from build123d import *

# Parameters (mm, degrees)
ESBO_O1_W                  = 90
ESBO_O1_H                  = 90
ESBO_O1_W_2                = 84
ESBO_O1_H_2                = 84
EXTRUS_O_FINA2_DEPTH       = 45
CORTE_EXTRUS_O1_DEPTH      = 78.942286341
CORTE_EXTRUS_O1_DEPTH_BACK = 78.942286341
ESBO_O5_W                  = 3
ESBO_O5_H                  = 84
ESBO_O7_R                  = 45
ESBO_O7_R_2                = 42
EXTRUS_O_FINA4_DEPTH       = 45
CORTE_EXTRUS_O2_DEPTH      = 111.227038425
CORTE_EXTRUS_O2_DEPTH_BACK = 111.227038425
ESBO_O9_W                  = 3
ESBO_O9_H                  = 45
RESSALTO_EXTRUS_O1_DEPTH   = 45
ESBO_O10_W                 = 3
ESBO_O10_H                 = 90
RESSALTO_EXTRUS_O2_DEPTH   = 45
ESBO_O11_W                 = 3
ESBO_O11_H                 = 90
RESSALTO_EXTRUS_O3_DEPTH   = 45
CORTE_EXTRUS_O4_DEPTH      = 78.942286341
CORTE_EXTRUS_O4_DEPTH_BACK = 78.942286341
CORTE_EXTRUS_O5_DEPTH      = 78.942286341
CORTE_EXTRUS_O5_DEPTH_BACK = 78.942286341
ESBO_O14_R                 = 42
CORTE_EXTRUS_O6_DEPTH      = 78.942286341
CORTE_EXTRUS_O6_DEPTH_BACK = 78.942286341
ESBO_O16_W                 = 84
ESBO_O16_H                 = 42
CORTE_EXTRUS_O8_DEPTH      = 78.942286341


with BuildPart() as part:
    # Esboço1 → Extrusão-Fina2 (new, symmetric)
    with BuildSketch(Plane(origin=(0, 0, 0), x_dir=(0, 0, -1), z_dir=(1, 0, 0))):
        Rectangle(ESBO_O1_W, ESBO_O1_H)
        Rectangle(ESBO_O1_W_2, ESBO_O1_H_2, mode=Mode.SUBTRACT)
    extrude(amount=EXTRUS_O_FINA2_DEPTH, both=True)

    # Esboço5 → Corte-extrusão1 (cut, two sides: drawn at the far end of the back side and taken through both)
    with BuildSketch(Plane(origin=(0, 0, 0), x_dir=(0, 0, -1), z_dir=(1, 0, 0)).offset(-CORTE_EXTRUS_O1_DEPTH_BACK)):
        with Locations((-43.5, 0)):
            Rectangle(ESBO_O5_W, ESBO_O5_H)
    extrude(amount=CORTE_EXTRUS_O1_DEPTH + CORTE_EXTRUS_O1_DEPTH_BACK, mode=Mode.SUBTRACT)

    # Esboço7 → Extrusão-Fina4 (add, symmetric)
    with BuildSketch(Plane(origin=(0, 0, 0), x_dir=(0, 0, -1), z_dir=(1, 0, 0))):
        with Locations((-45, 0)):
            Circle(ESBO_O7_R)
        with Locations((-45, 0)):
            Circle(ESBO_O7_R_2, mode=Mode.SUBTRACT)
    extrude(amount=EXTRUS_O_FINA4_DEPTH, both=True)

    # Esboço8 → Corte-extrusão2 (cut, two sides: drawn at the far end of the back side and taken through both)
    with BuildSketch(Plane(origin=(0, 0, 0), x_dir=(0, 0, -1), z_dir=(1, 0, 0)).offset(-CORTE_EXTRUS_O2_DEPTH_BACK)):
        Polygon((-45, -45), (-29.921616549, -39.200030007), (-3, 0), (-3, 45), (-95.371690307, 45), (-95.371690307, -45), align=None)
    extrude(amount=CORTE_EXTRUS_O2_DEPTH + CORTE_EXTRUS_O2_DEPTH_BACK, mode=Mode.SUBTRACT)

    # Esboço9 → Ressalto-extrusão1 (add, symmetric)
    with BuildSketch(Plane(origin=(0, 0, 0), x_dir=(0, 0, -1), z_dir=(1, 0, 0))):
        with Locations((-1.5, 22.5)):
            Rectangle(ESBO_O9_W, ESBO_O9_H)
    extrude(amount=RESSALTO_EXTRUS_O1_DEPTH, both=True)

    # Esboço10 → Ressalto-extrusão2 (add, symmetric)
    with BuildSketch(Plane(origin=(0, 0, 0), x_dir=(1, 0, 0), z_dir=(0, 1, 0))):
        with Locations((-43.5, 0)):
            Rectangle(ESBO_O10_W, ESBO_O10_H)
    extrude(amount=RESSALTO_EXTRUS_O2_DEPTH, both=True)

    # Esboço11 → Ressalto-extrusão3 (add, symmetric)
    with BuildSketch(Plane(origin=(0, 0, 0), x_dir=(1, 0, 0), z_dir=(0, 1, 0))):
        with Locations((43.5, 0)):
            Rectangle(ESBO_O11_W, ESBO_O11_H)
    extrude(amount=RESSALTO_EXTRUS_O3_DEPTH, both=True)

    # Esboço13 → Corte-extrusão4 (cut, two sides: drawn at the far end of the back side and taken through both)
    with BuildSketch(Plane(origin=(0, 0, 0), x_dir=(0, 0, -1), z_dir=(1, 0, 0)).offset(-CORTE_EXTRUS_O4_DEPTH_BACK)):
        Polygon((-3, 0), (-3, 45), (-45, 45), (-45, -45), align=None)
    extrude(amount=CORTE_EXTRUS_O4_DEPTH + CORTE_EXTRUS_O4_DEPTH_BACK, mode=Mode.SUBTRACT)

    # Esboço14 → Corte-extrusão5 (cut, two sides: drawn at the far end of the back side and taken through both)
    with BuildSketch(Plane(origin=(0, 0, 0), x_dir=(0, 0, -1), z_dir=(1, 0, 0)).offset(-CORTE_EXTRUS_O5_DEPTH_BACK)):
        with Locations((-45, 0)):
            Circle(ESBO_O14_R)
    extrude(amount=CORTE_EXTRUS_O5_DEPTH + CORTE_EXTRUS_O5_DEPTH_BACK, mode=Mode.SUBTRACT)

    # Esboço15 → Corte-extrusão6 (cut, two sides: drawn at the far end of the back side and taken through both)
    with BuildSketch(Plane(origin=(0, 0, 0), x_dir=(0, 0, -1), z_dir=(1, 0, 0)).offset(-CORTE_EXTRUS_O6_DEPTH_BACK)):
        Polygon((-45, -45), (-29.921616549, -39.200030007), (-45.529383671, 1.376024306), align=None)
    extrude(amount=CORTE_EXTRUS_O6_DEPTH + CORTE_EXTRUS_O6_DEPTH_BACK, mode=Mode.SUBTRACT)

    # Esboço16 → Corte-extrusão8 (cut, through all)
    with BuildSketch(Plane(origin=(0, 0, 0), x_dir=(1, 0, 0), z_dir=(0, 1, 0))):
        with Locations((0, 21)):
            Rectangle(ESBO_O16_W, ESBO_O16_H)
    extrude(amount=CORTE_EXTRUS_O8_DEPTH, mode=Mode.SUBTRACT)


solid = part.part
Geometry check sheet. Reference: the model listing, model coordinates, mm. A direction names the side the tool comes from. Round coordinates to 2 decimals unless told otherwise and drop trailing zeros. Loops run counter-clockwise (first coordinate to the right, second up) from the corner with the lowest first, then second, coordinate; pieces in that order, holes last.
Item 1: Thickness scan on line 1 (Z direction, x = -2, y = 41.5); line 2 (X direction, y = 41, z = -37); line 3 (Y direction, x = -3, z = 28). Record the ranges inside material, lowest first.
Item 2: Mould release check, pull along Z, two halves, no side actions. Record for faces 4 (the flat face through (-3.5, 45, 0.2)), 5 (the flat face through (-1, -42, -6)), 6 (the flat face through (-42, 1, -22)), 7 (the flat face through (-0.63, -42.14, 37.57)): pulls with the +Z half, pulls with the -Z half, needs draft (parallel to the pull), parting line crosses it, or undercut.
Item 3: Cross-section at C-C on z = -7.5. Record the boundary of the cut face in (x, y), then the cut area to 3 significant figures.
Item 4: Cross-section at A-A on y = 38. Record the boundary of the cut face in (x, z), then the cut area to 3 significant figures.
Item 5: Cross-section at B-B on z = 18.5. Record the boundary of the cut face in (x, y).
Item 6: Cross-section at D-D on x = 13. Record the boundary of the cut face in (y, z), then the cut area to 3 significant figures.
Item 7: Gauge pin test, flat ends, axial feed: pin 1 (3 mm diameter, centred on x = 4.5, z = 22.5, fed in from +Y); pin 2 (6 mm diameter, centred on x = 18, z = 27, fed in from +Y); pin 3 (1.5 mm diameter, centred on x = -18.5, z = -22, fed in from +Y); pin 4 (12 mm diameter, centred on y = -31.5, z = 27.5, fed in from +X). Record the tip position at first contact, or that the pin passes through.
Item 8: Access from +Z, -Z, +X, -X, +Y, -Y to the whole of each face (thin tool, end or side, straight path). Record for faces 1 (the cylindrical face through (0.588, -25.787, 8.121)), 2 (the flat face through (-1, 22, 3)), 3 (the flat face through (-1, 1, -42)).
Answer sheet:
1. line 1: z = -45 to -42, 0 to 3
1. line 2: x = -45 to -42, 42 to 45
1. line 3: y = -45 to -42, -41.67 to -38.41
2. face 4: needs draft
2. face 5: undercut
2. face 6: undercut
2. face 7: pulls with the +Z half
3. outline: (-45, -45) - (45, -45) - (45, 45) - (42, 45) - (42, -42) - (-42, -42) - (-42, 45) - (-45, 45) - close
3. area: 792 mm2
4. outline: (-45, -45) - (45, -45) - (45, 3) - (-45, 3) - close; hole (-42, -42) - (42, -42) - (42, 0) - (-42, 0) - close
4. area: 792 mm2
5. outline: (-45, -45) - (45, -45) - (45, -32.58) - (-45, -32.58) - close; hole (-42, -42) - (42, -42) - (42, -36.37) - (-42, -36.37) - close
6. outline: (-45, -45) - (45, -45) - (45, -42) - (-42, -42) - (-42, 28.84) arc R45 ccw to (0, 0) - (45, 0) - (45, 3) - (0, 3) arc R42 cw to (-39.2, 29.92) - (-45, 45) - close
6. area: 823 mm2
7. pin 1: stops at y = -34.47
7. pin 2: stops at y = -36.37
7. pin 3: stops at y = -42
7. pin 4: stops at x = 45
8. face 1: none
8. face 2: +Z, +X, -X, +Y
8. face 3: +Y
